The listing builds one solid part. Answer for the finished solid, in the listing's coordinates (mm). Face numbers are marked on the shaded views. A direction names the side the tool comes from. Round coordinates to 2 decimals unless told otherwise and drop trailing zeros. Write each loop counter-clockwise with the first axis right and the second up, starting at its lowest first coordinate (ties: lowest second). Pieces come first, ordered by that corner, then holes. Notation, with made-up numbers: M -24,56.5 L 4,56.5 A33 cw 4,85.5 Z; hole C -36,-18.75 d4. An arc over 180 degrees is marked long. Put each result on its own line as item: value. Start each with the question number.
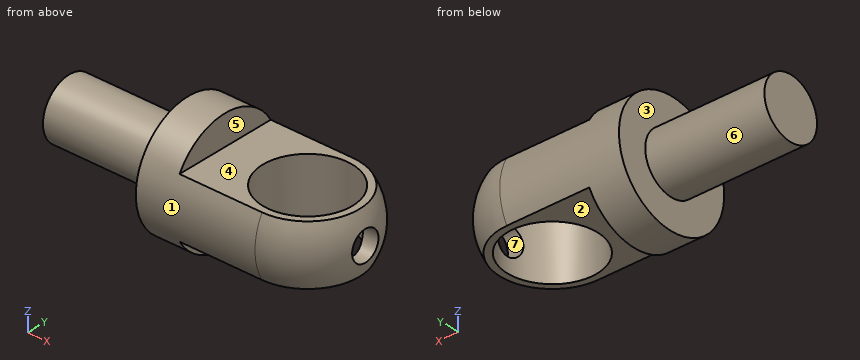
Autodesk Inventor part; units mm, degrees
ref_plane "Work Plane2" through (0, 4, 0) normal (0, 1, 0) x (-1, 0, 0)
ref_plane "Work Plane3" through (20, 0, 0) normal (1, 0, 0) x (0, 1, 0)
ref_plane "XY Plane" through (0, 0, 0) normal (0, 0, 1) x (1, 0, 0)
sketch "Sketch1" plane through (0, 0, 0) normal (0, 0, 1) x (1, 0, 0)
  line L0 (0, 0) -> (0, 2)
  line L1 (0, 2) -> (8, 2)
  line L2 (8, 2) -> (8, 4)
  line L3 (8, 4) -> (16, 4)
  arc A0 (20, 0) -> (16, 4) centre (16, 0) ccw
  line L4 (20, 0) -> (0, 0)
  dimension "d0" = 4
  dimension "d1" = 8
  dimension "d2" = 8
  dimension "d3" = 4
  dimension "d4" = 8
revolve "Revolution1" add sketch "Sketch1" angle 360 about axis through (20, 0, 0) along (-1, 0, 0)
thread "Thread1"
ref_plane "Work Plane2" through (0, 4, 0) normal (0, 1, 0) x (-1, 0, 0)
sketch "Sketch3" plane through (0, 4, 0) normal (0, 1, 0) x (-1, 0, 0)
  arc A0 (-16, 4) -> (-16, -4) centre (-16, 0) ccw
  line L0 (-16, -4) -> (-8, -4)
  line L1 (-8, -4) -> (-8, 4)
  line L2 (-16, 4) -> (-8, 4)
  line L3 (-19.4641, -2) -> (-10.4641, -2)
  line L4 (-10.4641, -2) -> (-10.4641, -4)
  line L5 (-19.4641, 2) -> (-10.4641, 2)
  line L6 (-10.4641, 2) -> (-10.4641, 4)
  point P0 (0, 0)
  dimension "d10" = 9
  dimension "d11" = 4
  dimension "d12" = 2
extrude "Extrusion1" cut sketch "Sketch3" against normal blind 8 contours L2 L6 L5 A0 | L3 L4 L0 A0
sketch "Sketch4" plane through (10.4641, -3.4641, 2) normal (0, 0, 1) x (1, 0, 0)
  arc A0 (5.5359, 0) -> (5.5359, 6.9282) centre (5.5359, 3.4641) ccw
  point P0 (-10.4641, 3.4641)
  point P1 (5.5359, 3.4641)
hole "Hole1" at (16, 0, 2) direction (0, 0, -1) diameter 6 depth 4
ref_plane "Work Plane3" through (20, 0, 0) normal (1, 0, 0) x (0, 1, 0)
sketch "Sketch5" plane through (20, 0, 0) normal (1, 0, 0) x (0, 1, 0)
  point P0 (0, 0)
  point P1 (0, 0)
hole "Hole2" at (20, 0, 0) direction (-1, 0, 0) diameter 2 depth 2.5
equation "\"d12\" = 0.5 * d11"
properties part number "9"
Item 1: Determine the mould class of the marked faces 4, 5, 6 and 7 for opening direction Z: released by +Z, released by -Z, zero draft, split by the parting line, or undercut.
Item 2: Section C-C (y = 2.25) is taken. Give the vertices of the cut face in (x, z).
Item 3: Flat-ended cylindrical pins translate along their axes: pin 1 (3.5 mm diameter, centred on x = 13, y = 0, fed in from -Z); pin 2 (4 mm diameter, centred on x = 12, y = 3, fed in from -Z); pin 3 (2 mm diameter, centred on y = 1, z = -2.5, fed in from +X). Find the tip coordinate at first contact, or state that the pin passes through.
Item 4: Consider line 1 along Z through (x, y) = (19.15, 0); line 2 along Y through (x, z) = (16, 0); line 3 along X through (y, z) = (-1.25, 3). Determine where each line is inside the solid, lowest interval first. Write a range as [from, to].
Item 5: Section B-B (x = 16.5) is taken. Give the vertices of the cut face in (y, z), and give its area (3 significant figures).
Item 6: Section D-D (z = 1.75) is taken. Give the vertices of the cut face in (x, y), and give its area (3 significant figures).
Item 7: Which of the six approach directions +Z, -Z, +X, -X, +Y, -Y give full straight-line access (tool end or side, diameter ignored) to the marked faces 1, 2 and 3?
Item 8: Section A-A (z = 0) is taken. Give the vertices of the cut face in (x, y).
Output values:
1. face 4: released by +Z
1. face 5: zero draft
1. face 6: split by the parting line
1. face 7: undercut
2. outline: M 8,-3.31 L 10.46,-3.31 L 10.46,-2 L 14.02,-2 L 14.02,2 L 10.46,2 L 10.46,3.31 L 8,3.31 Z; M 17.98,-2 L 18.63,-2 A3.31 ccw 18.63,2 L 17.98,2 Z
3. pin 1: stops at z = -2
3. pin 2: stops at z = -3.61
3. pin 3: stops at x = 19.62
4. line 1: z = [-2, -1], [1, 2]
4. line 2: y = [-4, -3], [3, 4]
4. line 3: x = [8, 10.46]
5. outline: M -3.43,-2 L -2.96,-2 L -2.96,2 L -3.43,2 A3.97 ccw Z; M 2.96,-2 L 3.43,-2 A3.97 ccw 3.43,2 L 2.96,2 Z
5. area: 6.68 mm^2
6. outline: M 0,-0.97 L 8,-0.97 L 8,-3.6 L 16,-3.6 A3.6 ccw 16,3.6 L 8,3.6 L 8,0.97 L 0,0.97 Z; hole C 16,0 d6
6. area: 65.1 mm^2
7. face 1: +X, -X
7. face 2: -Z, +X, +Y, -Y
7. face 3: -X
8. outline: M 0,-2 L 8,-2 L 8,-4 L 16,-4 A4 ccw 19.87,-1 L 18.83,-1 A3 cw long 18.83,1 L 19.87,1 A4 ccw 16,4 L 8,4 L 8,2 L 0,2 Z
